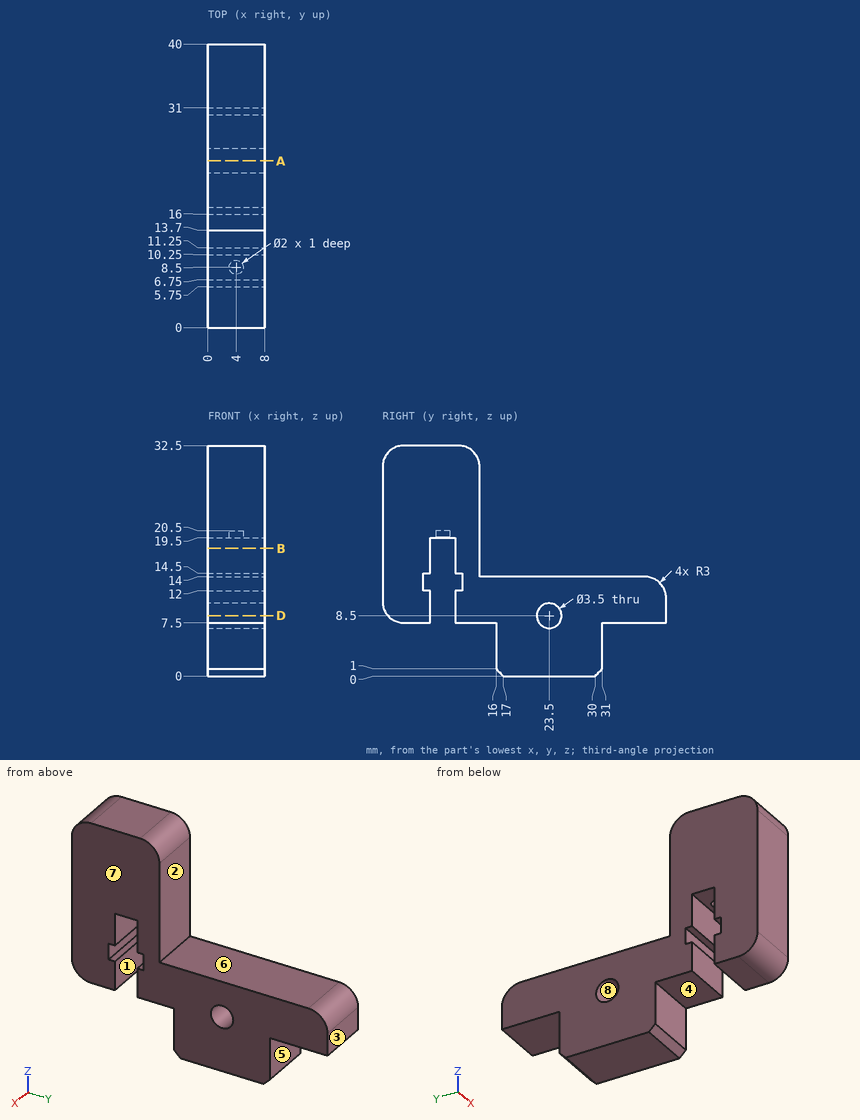
Geometry: see drawing. Coordinates: mm, zero at the bounding-box minimum. A direction names the side the tool comes from. Coordinates: 2 decimals unless noted, no trailing zeros. Loops run counter-clockwise (first coordinate to the right, second up) from the corner with the lowest first, then second, coordinate; pieces in that order, holes last. Notation, with made-up numbers: (52, 1) - (65, 1) arc R34 cw to (65, 38) - close; hole circle Ø9 at (-35.75, 18). An arc over 180 degrees is marked (long way). Put each result on its own line as item: value. Start each with the question number.
Q1. Pull-direction query (Z, two-part tool) for the marked faces 6, 7 and 8; classes: released by +Z, released by -Z, zero draft, split by the parting line, or undercut.
Q2. Cut plane B-B, the plane z = 18. Return loops of the section in (x, y).
Q3. Set-up query: the marked faces 1, 2, 3, 4 and 5. Return all of +Z, -Z, +X, -X, +Y, -Y with unobstructed straight access to the full face (end or side cutting, diameter ignored); none if empty.
Q4. Line query: line 1 (Y direction, x = 4, z = 19.95); line 2 (Y direction, x = 7.75, z = 17); line 3 (Y direction, x = 6, z = 8.5). Output: solid intervals per line, ascending.
Q5. Pin query (flat end, axial travel): pin 1 Ø1 at (x, y) = (5, 8.5) entering from -Z; pin 2 Ø10 at (y, z) = (34, 23.5) entering from -X; pin 3 Ø3 at (x, y) = (5.5, 13.5) entering from -Z; pin 4 Ø2 at (x, z) = (1, 9.5) entering from -Y. Return the tip coordinate at first contact, or that it passes through.
Q6. Cut plane A-A, the plane y = 23.5. Return loops of the section in (x, z).
Q7. Cut plane D-D, the plane z = 8.5. Return loops of the section in (x, y).
Filled sheet:
1. face 6: released by +Z
1. face 7: zero draft
1. face 8: undercut
2. outline: (0, 0) - (8, 0) - (8, 6.75) - (0, 6.75) - close; (0, 10.25) - (8, 10.25) - (8, 13.7) - (0, 13.7) - close
3. face 1: -Z, +X, -X
3. face 2: +Z, +X, -X, +Y
3. face 3: +Z, -Z, +X, -X, +Y
3. face 4: -Z, +X, -X, -Y
3. face 5: -Z, +X, -X, +Y
4. line 1: 0 to 7.5, 9.5 to 13.7
4. line 2: 0 to 6.75, 10.25 to 13.7
4. line 3: 0.76 to 6.75, 10.25 to 21.75, 25.25 to 40
5. pin 1: z = 19.5
5. pin 2: through
5. pin 3: z = 7.5
5. pin 4: y = 0
6. outline: (0, 0) - (8, 0) - (8, 6.75) - (0, 6.75) - close; (0, 10.25) - (8, 10.25) - (8, 14) - (0, 14) - close
7. outline: (0, 0.76) - (8, 0.76) - (8, 6.75) - (0, 6.75) - close; (0, 10.25) - (8, 10.25) - (8, 21.75) - (0, 21.75) - close; (0, 25.25) - (8, 25.25) - (8, 40) - (0, 40) - close
